```python
from build123d import *

# Parameters (mm, degrees)
BOSS_EXTRUDE1_DEPTH = 10
SKETCH3_W           = 75
SKETCH3_H           = 3
BOSS_EXTRUDE2_DEPTH = 6.5
SKETCH4_R           = 3
CUT_EXTRUDE2_DEPTH  = 10
SKETCH5_W           = 26
SKETCH5_H           = 14
BOSS_EXTRUDE3_DEPTH = 60
BOSS_EXTRUDE5_DEPTH = 4
CUT_EXTRUDE3_DEPTH  = 186.569394028
FILLET2_START       = -10
FILLET2_DEPTH       = 10
FILLET2_2_DEPTH     = 75
FILLET2_START_2     = -11
FILLET2_3_DEPTH     = 18
CUT_EXTRUDE4_DEPTH  = 187.815416923
FILLET3_R           = 1.25


with BuildPart() as part:
    # Sketch2 → Boss-Extrude1 (new body)
    with BuildSketch(Plane.XY):
        Polygon((0, 0), (130, 0), (130, 14), (75, 69), (75, 120), (0, 120), align=None)
    extrude(amount=-BOSS_EXTRUDE1_DEPTH)

    # Sketch3 → Boss-Extrude2 (add)
    with BuildSketch(Plane.XY):
        with Locations((37.5, 118.5)):
            Rectangle(SKETCH3_W, SKETCH3_H)
        with Locations((37.5, 79.5)):
            Rectangle(SKETCH3_W, SKETCH3_H)
    extrude(amount=BOSS_EXTRUDE2_DEPTH)

    # Sketch4 → Cut-Extrude2 (cut)
    with BuildSketch(Plane.XY):
        with Locations((10, 99)):
            Circle(SKETCH4_R)
        with Locations((65, 99)):
            Circle(SKETCH4_R)
    extrude(amount=-CUT_EXTRUDE2_DEPTH, mode=Mode.SUBTRACT)

    # Sketch5 → Boss-Extrude3 (add)
    with BuildSketch(Plane.XY):
        with Locations((117, 7)):
            Rectangle(SKETCH5_W, SKETCH5_H)
        with Locations((21, 7)):
            Rectangle(SKETCH5_W, SKETCH5_H)
    extrude(amount=BOSS_EXTRUDE3_DEPTH)

    # Sketch7 → Boss-Extrude5 (add)
    with BuildSketch(Plane.XY):
        with BuildLine():
            Line((53, 13), (53, 60))
            ThreePointArc((53, 60), (60, 67), (67, 60))
            Line((67, 60), (67, 13))
            ThreePointArc((67, 13), (60, 6), (53, 13))
        make_face()
    extrude(amount=BOSS_EXTRUDE5_DEPTH)

    # Sketch8 → Cut-Extrude3 (cut, through all)
    with BuildSketch(Plane.XY.offset(4)):
        with BuildLine():
            Line((62.2, 13), (62.2, 60))
            ThreePointArc((62.2, 60), (60, 62.2), (57.8, 60))
            Line((57.8, 60), (57.8, 13))
            ThreePointArc((57.8, 13), (60, 10.8), (62.2, 13))
        make_face()
    extrude(amount=-CUT_EXTRUDE3_DEPTH, mode=Mode.SUBTRACT)

    # Fillet2: read off the stored shape, not the designer's step
    # Fillet2 outline → Fillet2 (add)
    with BuildSketch(Plane.XY.offset(FILLET2_START)):
        with BuildLine():
            ThreePointArc((75.878679656, 68.121320344), (75.228361402, 69.09459039), (75, 70.242640687))
            Line((75, 70.242640687), (75, 69))
            Line((75, 69), (75.878679656, 68.121320344))
        make_face()
    extrude(amount=FILLET2_DEPTH)

    # Fillet2 2 outline → Fillet2 2 (add)
    with BuildSketch(Plane.YZ):
        with BuildLine():
            ThreePointArc((78, 3), (77.121320344, 0.878679656), (75, 0))
            Line((75, 0), (78, 0))
            Line((78, 0), (78, 3))
        make_face()
    extrude(amount=FILLET2_2_DEPTH)

    # Fillet2 3 outline → Fillet2 3 (cut)
    with BuildSketch(Plane.XY.offset(FILLET2_START_2)):
        with BuildLine():
            ThreePointArc((0, 117), (0.878679656, 119.121320344), (3, 120))
            Line((3, 120), (0, 120))
            Line((0, 120), (0, 117))
        make_face()
        with BuildLine():
            ThreePointArc((72, 120), (74.121320344, 119.121320344), (75, 117))
            Line((75, 117), (75, 120))
            Line((75, 120), (72, 120))
        make_face()
    extrude(amount=FILLET2_3_DEPTH, mode=Mode.SUBTRACT)

    # Sketch6 → Cut-Extrude4 (cut, through all)
    with BuildSketch(Plane.XY):
        Polygon((0, 13), (6, 7), (6, 25), (0, 19), align=None)
        Polygon((6, 47), (0, 53), (0, 59), (6, 65), align=None)
    extrude(amount=-CUT_EXTRUDE4_DEPTH, mode=Mode.SUBTRACT)

    # Fillet3
    fillet3_edges = [part.edges().sort_by_distance(p)[0] for p in [
        (0, 13, -5),
        (0, 19, -5),
        (6, 25, -5),
        (6, 7, -5),
        (6, 65, -5),
        (6, 47, -5),
        (0, 53, -5),
        (0, 59, -5),
    ]]
    fillet(fillet3_edges, radius=FILLET3_R)


solid = part.part
```
Source: CAD feature listing. Evaluate the final solid. Frame: model axes, mm. A direction names the side the tool comes from. Give positions to 0.01 mm unless a question says otherwise; leave off trailing zeros. Write each loop counter-clockwise with the first axis right and the second up, starting at its lowest first coordinate (ties: lowest second). Pieces come first, ordered by that corner, then holes.
1. First-contact query: pin 1 (12 mm diameter, centred on x = 54.5, y = 37.5, fed in from +Z); pin 2 (1.2 mm diameter, centred on y = 34.5, z = 3, fed in from -X); pin 3 (7 mm diameter, centred on x = 10, y = 99, fed in from -Z); pin 4 (5 mm diameter, centred on y = 57, z = -4.5, fed in from -X). Flat tips, straight axial feed; report the tip coordinate or a pass-through.
2. Section query A-A (y = 99). Return the cut outline in (x, z), then the cut area to 3 significant figures.
3. Section query B-B (z = 16). Return the cut outline in (x, y), then the cut area to 3 significant figures.
4. Material intervals for line 1 along Y through (x, z) = (10, -3); line 2 along Y through (x, z) = (21.5, 0.5); line 3 along X through (y, z) = (36, -6.5), sorted ascending.
5. Section query C-C (x = 65). Return the cut outline in (y, z).
6. Access query for faces 5 (the face through (37, 80, 6.5)), 6 (the face through (62.2, 36, -3)), 7 (the face through (37, 99, 0)). Directions: +Z, -Z, +X, -X, +Y, -Y. A direction counts if a zero-diameter tool reaches every point of the face in a straight line with its end or side. Return the directions, or none.
7. Section query D-D (x = 120). Return the cut outline in (y, z).
8. Pull-direction query (Y, two-part tool) for faces 1 (the face through (0.86, 119.1, -1.87)), 2 (the face through (8, 7, 30)), 3 (the face through (60, 62.2, -2.9)), 4 (the face through (37, 78, 5)); classes: +Y half, -Y half, draft (parallel to the pull), parting line (faces both ways), or undercut.
Output values:
1. pin 1: stops at z = 4
1. pin 2: stops at x = 53
1. pin 3: stops at z = -10
1. pin 4: stops at x = 6
2. outline: (0, -10) - (7, -10) - (7, 0) - (0, 0) - close; (13, -10) - (62, -10) - (62, 0) - (13, 0) - close; (68, -10) - (75, -10) - (75, 0) - (68, 0) - close
2. area: 630 mm2
3. outline: (8, 0) - (34, 0) - (34, 14) - (8, 14) - close; (104, 0) - (130, 0) - (130, 14) - (104, 14) - close
3. area: 728 mm2
4. line 1: y = 0 to 96, 102 to 120
4. line 2: y = 0 to 14, 76.66 to 81, 117 to 120
4. line 3: x = 0 to 57.8, 62.2 to 108
5. outline: (0, -10) - (96, -10) - (96, 0) - (81, 0) - (81, 6.5) - (78, 6.5) - (78, 3) arc R3 cw to (75, 0) - (64.9, 0) - (64.9, 4) - (8.1, 4) - (8.1, 0) - (0, 0) - close; (102, -10) - (120, -10) - (120, 6.5) - (117, 6.5) - (117, 0) - (102, 0) - close
6. face 5: +Z, +X, -X, +Y
6. face 6: +Z, -Z
6. face 7: +Z, +X, -X
7. outline: (0, -10) - (24, -10) - (24, 0) - (14, 0) - (14, 60) - (0, 60) - close
8. face 1: +Y half
8. face 2: draft
8. face 3: undercut
8. face 4: undercut
